```python
from build123d import *
from build123d.topology import SkipClean

# Parameters (mm, degrees)
BOSS_EXTRUDE1_DEPTH  = 15
SKETCH3_W            = 14
SKETCH3_H            = 18
BOSS_EXTRUDE2_DEPTH  = 150
BOSS_EXTRUDE3_DEPTH  = 18
SKETCH7_W            = 48
SKETCH7_H            = 46
SKETCH7_W_2          = 40
SKETCH7_H_2          = 38
BOSS_EXTRUDE4_DEPTH  = 10
BOSS_EXTRUDE5_DEPTH  = 18
FILLET2_R            = 10
CHAMFER2_SIZE        = 10
CHAMFER2_SIZE2       = 25.668100083
FILLET3_R            = 10
FILLET4_R            = 10
SKETCH11_W           = 40
SKETCH11_H           = 38
SKETCH11_W_2         = 34
SKETCH11_H_2         = 32
BOSS_EXTRUDE6_DEPTH  = 3
SKETCH12_W           = 32
SKETCH12_H           = 7
CUT_EXTRUDE2_DEPTH   = 5
CUT_EXTRUDE3_DEPTH   = 2
SKETCH15_R           = 5
BOSS_EXTRUDE8_DEPTH  = 14
BOSS_EXTRUDE10_DEPTH = 3


with BuildPart() as part:
    # Sketch1 → Boss-Extrude1 (new body)
    with BuildSketch(Plane(origin=(0, 0, 0), x_dir=(1, 0, 0), z_dir=(0, 1, 0))):
        with BuildLine():
            Line((35, -40), (-35, -40))
            ThreePointArc((-35, -40), (-45.606601718, -35.606601718), (-50, -25))
            Line((-50, -25), (-50, 25))
            ThreePointArc((-50, 25), (-45.606601718, 35.606601718), (-35, 40))
            Line((-35, 40), (35, 40))
            ThreePointArc((35, 40), (45.606601718, 35.606601718), (50, 25))
            Line((50, 25), (50, -25))
            ThreePointArc((50, -25), (45.606601718, -35.606601718), (35, -40))
        make_face()
    extrude(amount=BOSS_EXTRUDE1_DEPTH)

    # Sketch3 → Boss-Extrude2 (add)
    with BuildSketch(Plane(origin=(0, 15, 0), x_dir=(1, 0, 0), z_dir=(0, 1, 0))):
        with Locations((-43, 0)):
            Rectangle(SKETCH3_W, SKETCH3_H)
    extrude(amount=BOSS_EXTRUDE2_DEPTH)

    # Sketch5 → Boss-Extrude3 (add)
    with BuildSketch(Plane.XY.offset(9)):
        Polygon((-36, 15), (-36, 45), (-16, 15), align=None)
    extrude(amount=-BOSS_EXTRUDE3_DEPTH)



with BuildPart() as body_2:
    # Sketch7 → Boss-Extrude4 (new body)
    with BuildSketch(Plane(origin=(0, 175, 0), x_dir=(1, 0, 0), z_dir=(0, 1, 0))):
        with Locations((8, 0)):
            Rectangle(SKETCH7_W, SKETCH7_H)
        with Locations((8, 0)):
            Rectangle(SKETCH7_W_2, SKETCH7_H_2, mode=Mode.SUBTRACT)
    extrude(amount=-BOSS_EXTRUDE4_DEPTH)


with BuildPart() as part_1:
    add(part.part)

    add(body_2.part)  # Boss-Extrude5 merges body 2
    # Sketch8 → Boss-Extrude5 (add)
    with BuildSketch(Plane.XY.offset(9)):
        Polygon((-50, 165), (-16, 175), (-16, 165), (-36, 135.742522323), (-36, 165), align=None)
    extrude(amount=-BOSS_EXTRUDE5_DEPTH)

    # Fillet2
    # the kernel refuses this fillet: 10 mm, written as the material it adds along each edge
    with BuildSketch(Plane(origin=(-16, 165, 9), x_dir=(1, 0, 0), z_dir=(0, 0, -1))) as fillet2_piece_1:
        with BuildLine():
            CenterArc((5.338859158, 9.909967515), FILLET2_R, 214.35596202, 47.949835241)
            Line((-2.916615768, 4.266641036), (0, 0))
            Line((0, 0), (4, 0))
        make_face()
    extrude(amount=18)
    with BuildSketch(Plane(origin=(-36, 135.742522323, 9), x_dir=(0.5643326479831027, 0.825547492528673, 0), z_dir=(0, 0, -1))) as fillet2_piece_2:
        with BuildLine():
            CenterArc((FILLET2_R * 0.309130630834, FILLET2_R), FILLET2_R, 235.64403798, 34.35596202)
            Line((-FILLET2_R * 0.255202017149, FILLET2_R * 0.174452507471), (0, 0))
            Line((0, 0), (FILLET2_R * 0.309130630834, 0))
        make_face()
    extrude(amount=18)

    # Chamfer2
    chamfer2_edges = [part_1.edges().sort_by_distance(p)[0] for p in [
        (-50, 165, 0),
    ]]
    chamfer2_side = [part_1.faces().sort_by_distance(p)[0] for p in [
        (-33, 170, 0),
    ]]
    chamfer(chamfer2_edges, length=CHAMFER2_SIZE, length2=CHAMFER2_SIZE2, reference=chamfer2_side[0])

    # Fillet3
    fillet3_edges = [part_1.edges().sort_by_distance(p)[0] for p in [
        (-50, 139.331899917, 0),
        (-40.406344984, 167.82166324, 0),
    ]]
    fillet(fillet3_edges, radius=FILLET3_R)

    # Fillet4
    fillet4_edges = [part_1.edges().sort_by_distance(p)[0] for p in [
        (-36, 45, 0),
    ]]
    fillet(fillet4_edges, radius=FILLET4_R)

    # Sketch11 → Boss-Extrude6 (add)
    with BuildSketch(Plane.XZ.offset(-165)):
        with Locations((8, 0)):
            Rectangle(SKETCH11_W, SKETCH11_H)
        with Locations((8, 0)):
            Rectangle(SKETCH11_W_2, SKETCH11_H_2, mode=Mode.SUBTRACT)
    extrude(amount=-BOSS_EXTRUDE6_DEPTH)

    # Sketch12 → Cut-Extrude2 (cut)
    with BuildSketch(Plane(origin=(32, 0, 0), x_dir=(0, 0, -1), z_dir=(1, 0, 0))):
        with Locations((0, 171.5)):
            Rectangle(SKETCH12_W, SKETCH12_H)
    extrude(amount=-CUT_EXTRUDE2_DEPTH, mode=Mode.SUBTRACT)

    # Sketch13 → Cut-Extrude3 (cut)
    with BuildSketch(Plane(origin=(0, 15, 0), x_dir=(1, 0, 0), z_dir=(0, 1, 0))):
        with BuildLine():
            Line((-47, 12), (-13, 12))
            Line((-13, 12), (-13, -12))
            Line((-13, -12), (-47, -12))
            Line((-47, -12), (-47, -25))
            ThreePointArc((-47, -25), (-43.485281374, -33.485281374), (-35, -37))
            Line((-35, -37), (35, -37))
            ThreePointArc((35, -37), (43.485281374, -33.485281374), (47, -25))
            Line((47, -25), (47, 25))
            ThreePointArc((47, 25), (43.485281374, 33.485281374), (35, 37))
            Line((35, 37), (-35, 37))
            ThreePointArc((-35, 37), (-43.485281374, 33.485281374), (-47, 25))
            Line((-47, 25), (-47, 12))
        make_face()
        with BuildLine():
            Line((-45, 14), (-11, 14))
            Line((-11, 14), (-11, -14))
            Line((-11, -14), (-45, -14))
            Line((-45, -14), (-45, -25))
            ThreePointArc((-45, -25), (-42.071067812, -32.071067812), (-35, -35))
            Line((-35, -35), (35, -35))
            ThreePointArc((35, -35), (42.071067812, -32.071067812), (45, -25))
            Line((45, -25), (45, 25))
            ThreePointArc((45, 25), (42.071067812, 32.071067812), (35, 35))
            Line((35, 35), (-35, 35))
            ThreePointArc((-35, 35), (-42.071067812, 32.071067812), (-45, 25))
            Line((-45, 25), (-45, 14))
        make_face(mode=Mode.SUBTRACT)
    extrude(amount=-CUT_EXTRUDE3_DEPTH, mode=Mode.SUBTRACT)

    # Sketch15 → Boss-Extrude8 (add)
    with BuildSketch(Plane.ZY.offset(50)):
        with Locations(Location((0, 125, 0), (0, 0, 180))):
            Circle(SKETCH15_R)
        with Locations(Location((0, 29, 0), (0, 0, 180))):
            Circle(SKETCH15_R)
    extrude(amount=BOSS_EXTRUDE8_DEPTH)

    # Sketch16 → Boss-Extrude10 (add)
    with SkipClean():  # the faces are left unmerged after this step: merging them gives an invalid solid
        with BuildSketch(Plane.ZY.offset(64)):
            with BuildLine():
                Line((-5, 125), (-5, 137))
                ThreePointArc((-5, 137), (0, 142), (5, 137))
                Line((5, 137), (5, 125))
                ThreePointArc((5, 125), (0, 120), (-5, 125))
            make_face()
            with BuildLine():
                Line((-5, 17), (-5, 29))
                ThreePointArc((-5, 29), (0, 34), (5, 29))
                Line((5, 29), (5, 17))
                ThreePointArc((5, 17), (0, 12), (-5, 17))
            make_face()
        extrude(amount=BOSS_EXTRUDE10_DEPTH)
    add(part_1.part.scale(1), mode=Mode.REPLACE)  # the faces are merged on a copy


solid = part_1.part
```
Source: CAD feature listing. Evaluate the final solid. Frame: model axes, mm. A direction names the side the tool comes from. Round coordinates to 2 decimals unless told otherwise and drop trailing zeros. Loops run counter-clockwise (first coordinate to the right, second up) from the corner with the lowest first, then second, coordinate; pieces in that order, holes last.
1. Section query C-C on z = -33. Output: boundary loops of the cut face in (x, y), and give its area (3 significant figures).
2. Section query A-A on y = 72. Output: boundary loops of the cut face in (x, z), and give its area (3 significant figures).
3. Contact query for flat-ended pins moving along their axis: pin 1 (3 mm diameter, centred on y = 23.5, z = 1, fed in from +X); pin 2 (8 mm diameter, centred on y = 131, z = 1.5, fed in from +X); pin 3 (9 mm diameter, centred on y = 78, z = -4, fed in from +X); pin 4 (3 mm diameter, centred on y = 53.5, z = -12, fed in from +X). Output: stop coordinate, or through.
4. Section query D-D on x = -59. Output: boundary loops of the cut face in (y, z).
5. Section query B-B on x = 39. Output: boundary loops of the cut face in (y, z), and give its area (3 significant figures).
6. Access query for faces 1 (the cylindrical face through (43.39, 14.01, 33.58)), 2 (the cylindrical face through (-65, 12, 0)), 3 (the flat face through (8, 170, -23)). Directions: +Z, -Z, +X, -X, +Y, -Y. A direction counts if a zero-diameter tool reaches every point of the face in a straight line with its end or side. Return the directions, or none.
7. Mould query, pull axis X, two halves, no side actions, for faces 4 (the cylindrical face through (-42.15, 14.01, 31.99)), 5 (the cylindrical face through (-65, 142, 0)), 6 (the flat face through (-16, 170, 16)), 7 (the cylindrical face through (43.58, 14.01, -33.39)). Classes: released by +X, released by -X, zero draft, split by the parting line, or undercut.
8. Ray query, L1, parallel to Y at x = 24, z = -22; L2, parallel to Y at x = 39.5, z = 17.5; L3, parallel to Z at x = -42.5, y = 63. Return the intervals inside material, ascending.
Answers below:
1. outline: (-47.69, 0) - (47.69, 0) - (47.69, 15) - (43.94, 15) - (43.94, 13) - (41, 13) - (41, 15) - (-41, 15) - (-41, 13) - (-43.94, 13) - (-43.94, 15) - (-47.69, 15) - close
1. area: 1,420 mm2
2. outline: (-50, -9) - (-36, -9) - (-36, 9) - (-50, 9) - close
2. area: 252 mm2
3. pin 1: stops at x = -20.67
3. pin 2: stops at x = -35.72
3. pin 3: stops at x = -36
3. pin 4: passes through
4. outline: circle Ø10 at (29, 0); circle Ø10 at (125, 0)
5. outline: (0, -39.46) - (15, -39.46) - (15, -36.31) - (13, -36.31) - (13, -34.17) - (15, -34.17) - (15, 34.17) - (13, 34.17) - (13, 36.31) - (15, 36.31) - (15, 39.46) - (0, 39.46) - close
5. area: 1,180 mm2
6. face 1: +Y
6. face 2: -X, -Y
6. face 3: -Z, +X, -X, +Y
7. face 4: undercut
7. face 5: zero draft
7. face 6: released by -X
7. face 7: undercut
8. L1: y = 0 to 15, 165 to 175
8. L2: y = 0 to 15
8. L3: z = -9 to 9
